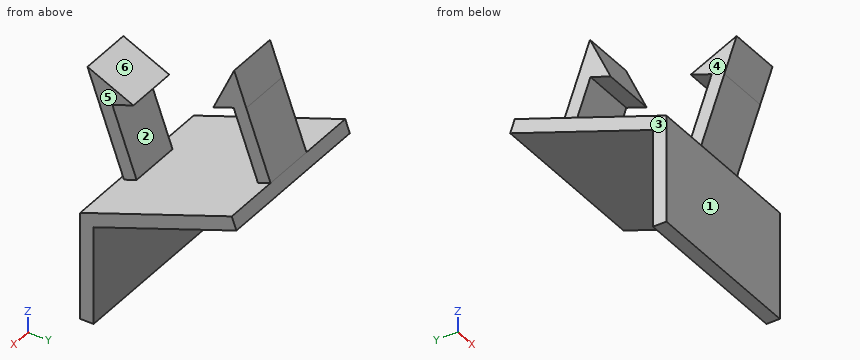
from build123d import *

# Parameters (mm, degrees)
SKETCH2_W           = 40.132
SKETCH2_H           = 25.4
BOSS_EXTRUDE1_DEPTH = 3.175
BOSS_EXTRUDE2_DEPTH = 40.132
SKETCH5_W           = 12.7
SKETCH5_H           = 3.175
BOSS_EXTRUDE3_DEPTH = 16.764
BOSS_EXTRUDE4_DEPTH = 12.7


with BuildPart() as part:
    # Sketch2 → Boss-Extrude1 (new body)
    with BuildSketch(Plane(origin=(0, 0, 0), x_dir=(1, 0, 0), z_dir=(0, 1, 0))):
        with Locations((-38.371824561, 11.620425731)):
            Rectangle(SKETCH2_W, SKETCH2_H)
    extrude(amount=BOSS_EXTRUDE1_DEPTH)

    # Sketch3 → Boss-Extrude2 (add)
    with BuildSketch(Plane(origin=(-18.305824561, 0, 0), x_dir=(0, 0, -1), z_dir=(1, 0, 0))):
        Polygon((-1.079574269, 0), (-14.11054173, 35.802288852), (-11.127017659, 36.888202807), (1.143584665, 3.175), align=None)
    extrude(amount=-BOSS_EXTRUDE2_DEPTH)

    # Sketch5 → Boss-Extrude3 (add)
    with BuildSketch(Plane(origin=(0, -0.346968482, 0.953288069), x_dir=(1, 0, 0), z_dir=(0, -0.34202014332566316, 0.9396926207859104))):
        with Locations((-38.371824561, 36.881736146)):
            Rectangle(SKETCH5_W, SKETCH5_H)
        with Locations((-38.371824561, 3.226736146)):
            Rectangle(SKETCH5_W, SKETCH5_H)
    extrude(amount=BOSS_EXTRUDE3_DEPTH)

    # Sketch6 → Boss-Extrude4 (add)
    with BuildSketch(Plane.ZY.offset(44.721824561)):
        Polygon((29.863548825, 30.068663169), (37.740052372, 27.201850328), (27.040172541, 22.311500585), align=None)
        Polygon((17.266946946, -4.540216054), (20.159821722, 3.407892071), (25.215055071, -7.433090831), align=None)
    extrude(amount=-BOSS_EXTRUDE4_DEPTH)


solid = part.part
Source: CAD feature listing. Evaluate the final solid. Frame: model axes, mm. Face numbers are marked on the shaded views. A direction names the side the tool comes from. Give positions to 0.01 mm unless a question says otherwise; leave off trailing zeros. Order: outer loops, then holes, each group sorted by start corner. A loop starts at its lowest first (then second) coordinate and runs counter-clockwise, first axis right, second up. Notation, with made-up numbers: (-37, 29.25) -> (2, 29.25) arc R6 ccw to (2, 39.25) -> close; hole circle Ø11 at (-26, 45). An arc over 180 degrees is marked (long way). Write item = value, one per line.
Q1. Material intervals for line 1 (Y direction, x = -36, z = -4.5) (3 decimals); line 2 (X direction, y = -1, z = 13.5); line 3 (Z direction, x = -36.5, y = 17), sorted ascending. Write a range as from..to.
Data:
line_1 = 0..3.175
line_2 = -44.72..-32.02
line_3 = 3.89..7.27
Q2. Set-up query: the marked faces 4, 5 and 6. Return all of +Z, -Z, +X, -X, +Y, -Y with unobstructed straight access to the full face (end or side cutting, diameter ignored); none if empty.
Data:
face_4 = +Z, -X, -Y
face_5 = +Z, +X, -Y
face_6 = +Z, +X, -X
Q3. Cut plane D-D, the plane z = -10. Output: boundary loops of the cut face in (x, y) (3 decimals), and give its area (3 significant figures).
Data:
outline = (-58.438, 0) -> (-18.306, 0) -> (-18.306, 3.175) -> (-58.438, 3.175) -> close
area = 127 mm^2
Q4. Pin query (flat end, axial travel): pin 1 (4 mm diameter, centred on y = 31, z = 22.5, fed in from -X); pin 2 (6 mm diameter, centred on x = -28, z = -15, fed in from +Y) (3 decimals); pin 3 (4 mm diameter, centred on x = -26.5, y = 21.5, fed in from -Z); pin 4 (6 mm diameter, centred on x = -51, z = 18.5, fed in from -Y). Return the tip coordinate at first contact, or that it passes through.
Data:
pin_1 = -44.72
pin_2 = 3.175
pin_3 = 4.8
pin_4 = through
Q5. Cut plane A-A, the plane z = 21.5. Output: boundary loops of the cut face in (x, y).
Data:
outline = (-44.72, -6.08) -> (-32.02, -6.08) -> (-32.02, 0.53) -> (-44.72, 0.53) -> close; (-44.72, 29.73) -> (-32.02, 29.73) -> (-32.02, 33.11) -> (-44.72, 33.11) -> close
Q6. Pull-direction query (Y, two-part tool) for the marked faces 1, 2 and 3; classes: released by +Y, released by -Y, zero draft, split by the parting line, or undercut.
Data:
face_1 = released by -Y
face_2 = undercut
face_3 = zero draft
Q7. Cut plane C-C, the plane x = -42.5. Output: boundary loops of the cut face in (y, z) (1 decimal), and give its area (3 significant figures).
Data:
outline = (-7.4, 25.2) -> (1.2, 1.5) -> (0, 1.1) -> (0, -24.3) -> (3.2, -24.3) -> (3.2, -1.1) -> (36.9, 11.1) -> (27.2, 37.7) -> (22.3, 27) -> (27.1, 28.8) -> (32.8, 13) -> (4.2, 2.6) -> (-1.6, 18.4) -> (3.4, 20.2) -> close
area = 371 mm^2
Q8. Cut plane B-B, the plane y = 26. Output: boundary loops of the cut face in (x, z), and give its area (3 significant figures).
Data:
outline = (-58.44, 7.16) -> (-18.31, 7.16) -> (-18.31, 10.54) -> (-58.44, 10.54) -> close; (-44.72, 28.38) -> (-32.02, 28.38) -> (-32.02, 35.11) -> (-44.72, 35.11) -> close
area = 221 mm^2
